Model file for the job. Use its own axes, mm. Give positions to 0.01 mm unless a question says otherwise; leave off trailing zeros. Order: outer loops, then holes, each group sorted by start corner. A loop starts at its lowest first (then second) coordinate and runs counter-clockwise, first axis right, second up. Notation, with made-up numbers: (17, -19.75) - (69, -19.75) arc R32 ccw to (69, 11.25) - close; hole circle Ø6 at (33.5, 44). An arc over 180 degrees is marked (long way). Use CSV: the item, a comma, the result in double quotes. Start each with the question number.
(1) Probe L1, parallel to Z at x = -25.4, y = 3.5; L2, parallel to Z at x = 99, y = 3.5; L3, parallel to X at y = 1.75, z = -9.14. List the from-to ranges inside material, lowest first.
(2) Band-saw the part on A-A, the plane z = 6.36. Give the cut face in (x, y).
(3) Band-saw the part on C-C, the plane y = 2.75. Count the separate pieces of the cut face and the enclosed holes in it, then the cut area to 3 significant figures.
(4) Band-saw the part on D-D, the plane x = -7.5. Give the cut face in (y, z), then the cut area to 3 significant figures.
(5) Band-saw the part on B-B, the plane x = 89.5. Give the cut face in (y, z).
(6) Drop flat-ended pins along their axis: pin 1 Ø2 at (x, z) = (105.57, -9.14) entering from -Y; pin 2 Ø1 at (x, y) = (65, 3) entering from -Z; pin 3 Ø3.5 at (x, y) = (18.5, 2) entering from +Z; pin 4 Ø1 at (y, z) = (4.5, 23) entering from -X. Give the stop position or say it passes through.
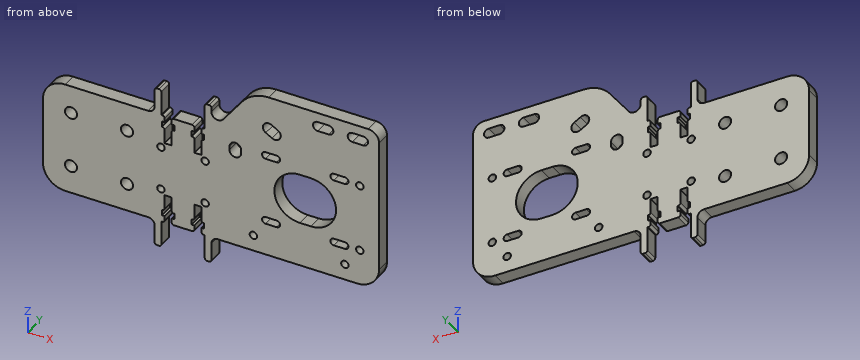
from build123d import *

# Parameters (mm, degrees)
BOSS_EXTRUDE1_DEPTH  = 6.35
M5_CLEARANCE_HOLE1_D = 5.5
M3_CLEARANCE_HOLE1_D = 3.4
CUT_EXTRUDE1_DEPTH   = 7.35
CUT_EXTRUDE2_DEPTH   = 7.35
FILLET1_R            = 10
CUT_EXTRUDE3_DEPTH   = 7.35
M3_CLEARANCE_HOLE2_D = 3.4
FILLET3_R            = 5
SKETCH13_W           = 3
SKETCH13_H           = 12
BOSS_EXTRUDE2_DEPTH  = 6.35
FILLET4_R            = 3
CUT_EXTRUDE4_DEPTH   = 7.35
FILLET5_R            = 1
FILLET6_R            = 1


with BuildPart() as part:
    # Sketch1 → Boss-Extrude1 (new body)
    with BuildSketch(Plane(origin=(0, 0, 0), x_dir=(1, 0, 0), z_dir=(0, 1, 0))):
        with BuildLine():
            Line((38.1, -25.4), (-38.1, -25.4))
            Line((-38.1, -25.4), (-38.1, 25.4))
            Line((-38.1, 25.4), (38.1, 25.4))
            Line((38.1, 25.4), (114.321209859, 25.4))
            Line((114.321209859, 25.4), (114.321209859, -50.04))
            Line((114.321209859, -50.04), (64.241941751, -50.04))
            ThreePointArc((64.241941751, -50.04), (57.570841587, -48.474895705), (52.291870426, -44.10618968))
            Line((52.291870426, -44.10618968), (38.1, -25.4))
        make_face()
    extrude(amount=BOSS_EXTRUDE1_DEPTH)

    # M5 Clearance Hole1 (through all)
    with Locations(Plane(origin=(0, 6.35, 0), x_dir=(1, 0, 0), z_dir=(0, 1, 0))):
        with Locations((-25.4, 12.7), (0, 12.7), (0, -12.7), (-25.4, -12.7)):
            Hole(M5_CLEARANCE_HOLE1_D / 2)

    # M3 Clearance Hole1 (through all)
    with Locations(Plane(origin=(0, 6.35, 0), x_dir=(1, 0, 0), z_dir=(0, 1, 0))):
        with Locations((15.4, 10), (35.4, 10), (35.4, -10), (15.4, -10)):
            Hole(M3_CLEARANCE_HOLE1_D / 2)

    # Sketch6 → Cut-Extrude1 (cut, through all)
    with BuildSketch(Plane(origin=(0, 6.35, 0), x_dir=(1, 0, 0), z_dir=(0, 1, 0))):
        with BuildLine():
            Line((62.821209859, 7.54), (67.821209859, 7.54))
            ThreePointArc((67.821209859, 7.54), (69.421209859, 9.14), (67.821209859, 10.74))
            Line((67.821209859, 10.74), (62.821209859, 10.74))
            ThreePointArc((62.821209859, 10.74), (61.221209859, 9.14), (62.821209859, 7.54))
        make_face()
        with BuildLine():
            Line((62.821209859, -23.46), (67.821209859, -23.46))
            ThreePointArc((67.821209859, -23.46), (69.421209859, -21.86), (67.821209859, -20.26))
            Line((67.821209859, -20.26), (62.821209859, -20.26))
            ThreePointArc((62.821209859, -20.26), (61.221209859, -21.86), (62.821209859, -23.46))
        make_face()
        with BuildLine():
            Line((93.821209859, -23.46), (98.821209859, -23.46))
            ThreePointArc((98.821209859, -23.46), (100.421209859, -21.86), (98.821209859, -20.26))
            Line((98.821209859, -20.26), (93.821209859, -20.26))
            ThreePointArc((93.821209859, -20.26), (92.221209859, -21.86), (93.821209859, -23.46))
        make_face()
        with BuildLine():
            Line((93.821209859, 7.54), (98.821209859, 7.54))
            ThreePointArc((98.821209859, 7.54), (100.421209859, 9.14), (98.821209859, 10.74))
            Line((98.821209859, 10.74), (93.821209859, 10.74))
            ThreePointArc((93.821209859, 10.74), (92.221209859, 9.14), (93.821209859, 7.54))
        make_face()
        with BuildLine():
            Line((78.321209859, -17.86), (83.321209859, -17.86))
            ThreePointArc((83.321209859, -17.86), (94.821209859, -6.36), (83.321209859, 5.14))
            Line((83.321209859, 5.14), (78.321209859, 5.14))
            ThreePointArc((78.321209859, 5.14), (66.821209859, -6.36), (78.321209859, -17.86))
        make_face()
    extrude(amount=-CUT_EXTRUDE1_DEPTH, mode=Mode.SUBTRACT)

    # Sketch7 → Cut-Extrude2 (cut, through all)
    with BuildSketch(Plane(origin=(0, 6.35, 0), x_dir=(1, 0, 0), z_dir=(0, 1, 0))):
        with BuildLine():
            Line((65.751764766, -31.105892862), (62.915452987, -32.745892862))
            ThreePointArc((62.915452987, -32.745892862), (61.947834614, -36.366488764), (65.568430515, -37.334107138))
            Line((65.568430515, -37.334107138), (68.404742294, -35.694107138))
            ThreePointArc((68.404742294, -35.694107138), (69.372360668, -32.073511236), (65.751764766, -31.105892862))
        make_face()
        with BuildLine():
            Line((46.45, -19.08), (46.45, -20.72))
            ThreePointArc((46.45, -20.72), (49.1, -23.37), (51.75, -20.72))
            Line((51.75, -20.72), (51.75, -19.08))
            ThreePointArc((51.75, -19.08), (49.1, -16.43), (46.45, -19.08))
        make_face()
    extrude(amount=-CUT_EXTRUDE2_DEPTH, mode=Mode.SUBTRACT)

    # Fillet1
    fillet1_edges = [part.edges().sort_by_distance(p)[0] for p in [
        (-38.1, 3.175, -25.4),
        (114.321209859, 3.175, -25.4),
        (-38.1, 3.175, 25.4),
    ]]
    fillet(fillet1_edges, radius=FILLET1_R)

    # Sketch8 → Cut-Extrude3 (cut, through all)
    with BuildSketch(Plane(origin=(0, 6.35, 0), x_dir=(1, 0, 0), z_dir=(0, 1, 0))):
        with BuildLine():
            Line((107.171209859, -41.46), (102.221209859, -41.46))
            ThreePointArc((102.221209859, -41.46), (100.071209859, -43.61), (102.221209859, -45.76))
            Line((102.221209859, -45.76), (107.171209859, -45.76))
            ThreePointArc((107.171209859, -45.76), (109.321209859, -43.61), (107.171209859, -41.46))
        make_face()
        with BuildLine():
            Line((86.471209859, -45.76), (91.421209859, -45.76))
            ThreePointArc((91.421209859, -45.76), (93.571209859, -43.61), (91.421209859, -41.46))
            Line((91.421209859, -41.46), (86.471209859, -41.46))
            ThreePointArc((86.471209859, -41.46), (84.321209859, -43.61), (86.471209859, -45.76))
        make_face()
    extrude(amount=-CUT_EXTRUDE3_DEPTH, mode=Mode.SUBTRACT)

    # M3 Clearance Hole2 (through all)
    with Locations(Plane(origin=(0, 6.35, 0), x_dir=(1, 0, 0), z_dir=(0, 1, 0))):
        with Locations((57.321209859, 18.14), (98.821209859, 18.14), (105.566578641, 9.14), (105.566578641, -21.61)):
            Hole(M3_CLEARANCE_HOLE2_D / 2)

    # Fillet3
    fillet3_edges = [part.edges().sort_by_distance(p)[0] for p in [
        (114.321209859, 3.175, 50.04),
    ]]
    fillet(fillet3_edges, radius=FILLET3_R)

    # Sketch13 → Boss-Extrude2 (add)
    with BuildSketch(Plane(origin=(0, 6.35, 0), x_dir=(1, 0, 0), z_dir=(0, 1, 0))):
        with Locations((36.75, 31.4)):
            Rectangle(SKETCH13_W, SKETCH13_H)
        with Locations((14.05, 31.4)):
            Rectangle(SKETCH13_W, SKETCH13_H)
        with Locations((14.05, -31.4)):
            Rectangle(SKETCH13_W, SKETCH13_H)
        with Locations((36.75, -31.4)):
            Rectangle(SKETCH13_W, SKETCH13_H)
    extrude(amount=-BOSS_EXTRUDE2_DEPTH)

    # Fillet4
    fillet4_edges = [part.edges().sort_by_distance(p)[0] for p in [
        (38.25, 3.175, -25.4),
        (12.55, 3.175, -25.4),
        (12.55, 3.175, 25.4),
        (38.25, 3.175, 25.597713787),
    ]]
    fillet(fillet4_edges, radius=FILLET4_R)

    # Sketch14 → Cut-Extrude4 (cut, through all)
    with BuildSketch(Plane(origin=(0, 6.35, 0), x_dir=(1, 0, 0), z_dir=(0, 1, 0))):
        Polygon((17.05, 12.4), (20.25, 12.4), (20.25, 19.8), (21.5, 19.8), (21.5, 22.4), (20.25, 22.4), (20.25, 25.4), (17.05, 25.4), (17.05, 22.4), (15.8, 22.4), (15.8, 19.8), (17.05, 19.8), align=None)
        Polygon((35, 22.4), (33.75, 22.4), (33.75, 25.4), (30.55, 25.4), (30.55, 22.4), (29.3, 22.4), (29.3, 19.8), (30.55, 19.8), (30.55, 12.4), (33.75, 12.4), (33.75, 19.8), (35, 19.8), align=None)
        Polygon((21.5, -22.4), (20.25, -22.4), (20.25, -25.4), (17.05, -25.4), (17.05, -22.4), (15.8, -22.4), (15.8, -19.8), (17.05, -19.8), (17.05, -12.4), (20.25, -12.4), (20.25, -19.8), (21.5, -19.8), align=None)
        Polygon((30.55, -19.8), (29.3, -19.8), (29.3, -22.4), (30.55, -22.4), (30.55, -25.4), (33.75, -25.4), (33.75, -22.4), (35, -22.4), (35, -19.8), (33.75, -19.8), (33.75, -12.4), (30.55, -12.4), align=None)
    extrude(amount=-CUT_EXTRUDE4_DEPTH, mode=Mode.SUBTRACT)

    # Fillet5
    fillet5_edges = [part.edges().sort_by_distance(p)[0] for p in [
        (35.25, 3.175, -37.4),
        (38.25, 3.175, -37.4),
        (12.55, 3.175, -37.4),
        (15.55, 3.175, -37.4),
        (15.55, 3.175, 37.4),
        (12.55, 3.175, 37.4),
        (38.25, 3.175, 37.4),
        (35.25, 3.175, 37.4),
        (20.25, 3.175, 25.4),
        (17.05, 3.175, 25.4),
        (17.05, 3.175, 19.8),
        (20.25, 3.175, 19.8),
        (30.55, 3.175, 19.8),
        (33.75, 3.175, 19.8),
        (33.75, 3.175, 25.4),
        (30.55, 3.175, 25.4),
    ]]
    fillet(fillet5_edges, radius=FILLET5_R)

    # Fillet6
    fillet6_edges = [part.edges().sort_by_distance(p)[0] for p in [
        (20.25, 3.175, -19.8),
        (17.05, 3.175, -19.8),
        (17.05, 3.175, -25.4),
        (20.25, 3.175, -25.4),
        (33.75, 3.175, -19.8),
        (30.55, 3.175, -19.8),
        (30.55, 3.175, -25.4),
        (33.75, 3.175, -25.4),
    ]]
    fillet(fillet6_edges, radius=FILLET6_R)


solid = part.part
Answer block:
1,L1,"z = -25.4 to -15.45, -9.95 to 9.95, 15.45 to 25.4"
1,L2,"z = -25.4 to -19.83, -16.45 to -10.73, -7.55 to 20.27, 23.45 to 50.04"
1,L3,"x = -38.1 to 13.93, 16.87 to 33.93, 36.87 to 61.22, 69.42 to 92.22, 100.42 to 103.87, 107.27 to 114.32"
2,outline,"(-38.1, 0) - (66.82, 0) - (66.82, 6.35) - (-38.1, 6.35) - close; (94.82, 0) - (114.32, 0) - (114.32, 6.35) - (94.82, 6.35) - close"
3,separate pieces,"1"
3,enclosed holes,"21"
3,area,"8,340 mm2"
4,outline,"(0, -25.4) - (6.35, -25.4) - (6.35, 25.4) - (0, 25.4) - close"
4,area,"323 mm2"
5,outline,"(0, -25.4) - (6.35, -25.4) - (6.35, -3.34) - (0, -3.34) - close; (0, 16.06) - (6.35, 16.06) - (6.35, 41.46) - (0, 41.46) - close; (0, 45.76) - (6.35, 45.76) - (6.35, 50.04) - (0, 50.04) - close"
6,pin 1,"passes through"
6,pin 2,"stops at z = -25.4"
6,pin 3,"stops at z = 25.11"
6,pin 4,"stops at x = -35.14"
